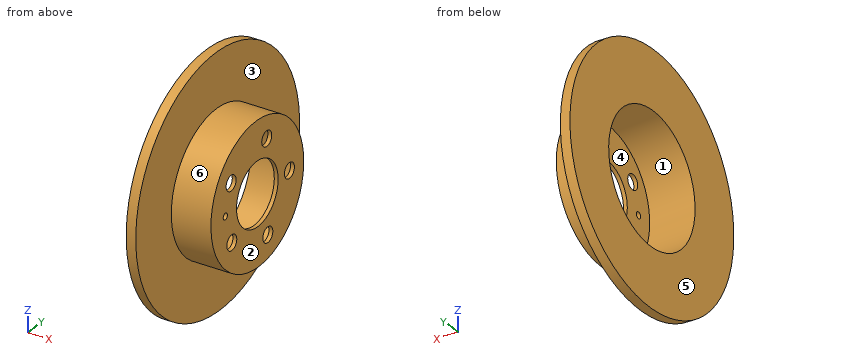
from build123d import *

# Parameters (mm, degrees)
SZKIC1_W                    = 10
SZKIC1_H                    = 128
SZKIC7_R                    = 72.5
DODANIE_WYCI_GNI_CIE1_DEPTH = 41.3
SZKIC8_R                    = 67.5
WYTNIJ_WYCI_GNI_CIE7_DEPTH  = 47.3
WYTNIJ_WYCI_GNI_CIE8_REACH  = 190.148
SZKIC9_R                    = 32.5
WYTNIJ_WYCI_GNI_CIE9_REACH  = 190.148
SZKIC10_R                   = 3.3
SZKIC10_R_2                 = 7.8


with BuildPart() as part:
    # Szkic1 → Obrót1 (revolve)
    with BuildSketch(Plane(origin=(0, 0, 0), x_dir=(1, 0, 0), z_dir=(0, 1, 0)), mode=Mode.PRIVATE) as obr_t1_sk:
        with Locations((5, 64)):
            Rectangle(SZKIC1_W, SZKIC1_H)
    revolve(obr_t1_sk.sketch.rotate(Axis((0, 0, 0), (1, 0, 0)), 180), axis=Axis((0, 0, 0), (1, 0, 0)))

    # Szkic7 → Dodanie-wyciągnięcie1 (add)
    with BuildSketch(Plane(origin=(10, 0, 0), x_dir=(0, 0, -1), z_dir=(1, 0, 0))):
        with Locations(Location((0, 0, 0), (0, 0, 180))):
            Circle(SZKIC7_R)
    extrude(amount=DODANIE_WYCI_GNI_CIE1_DEPTH)

    # Szkic8 → Wytnij-wyciągnięcie7 (cut)
    with BuildSketch(Plane.ZY):
        Circle(SZKIC8_R)
    extrude(amount=-WYTNIJ_WYCI_GNI_CIE7_DEPTH, mode=Mode.SUBTRACT)

    # Szkic9 → Wytnij-wyciągnięcie8 (cut, up to next)
    with BuildSketch(Plane(origin=(51.3, 0, 0), x_dir=(0, 0, -1), z_dir=(1, 0, 0)), mode=Mode.PRIVATE) as wytnij_wyci_gni_cie8_sk1:
        Circle(SZKIC9_R)
    wytnij_wyci_gni_cie8_tool1 = extrude(wytnij_wyci_gni_cie8_sk1.sketch, amount=-WYTNIJ_WYCI_GNI_CIE8_REACH, mode=Mode.PRIVATE) & part.part
    add(wytnij_wyci_gni_cie8_tool1.solids().sort_by_distance((51.3, 0, 0))[0], mode=Mode.SUBTRACT)

    # Szkic10 → Wytnij-wyciągnięcie9 (cut, up to next)
    with BuildSketch(Plane(origin=(51.3, 0, 0), x_dir=(0, 0, -1), z_dir=(1, 0, 0)), mode=Mode.PRIVATE) as wytnij_wyci_gni_cie9_sk1:
        with Locations((0, -50)):
            Circle(SZKIC10_R)
    wytnij_wyci_gni_cie9_tool1 = extrude(wytnij_wyci_gni_cie9_sk1.sketch, amount=-WYTNIJ_WYCI_GNI_CIE9_REACH, mode=Mode.PRIVATE) & part.part
    # Szkic10 → Wytnij-wyciągnięcie9 (cut, up to next)
    with BuildSketch(Plane(origin=(51.3, 0, 0), x_dir=(0, 0, -1), z_dir=(1, 0, 0)), mode=Mode.PRIVATE) as wytnij_wyci_gni_cie9_sk2:
        with Locations((-28.682618124, -40.95494375)):
            Circle(SZKIC10_R_2)
    wytnij_wyci_gni_cie9_tool2 = extrude(wytnij_wyci_gni_cie9_sk2.sketch, amount=-WYTNIJ_WYCI_GNI_CIE9_REACH, mode=Mode.PRIVATE) & part.part
    # Szkic10 → Wytnij-wyciągnięcie9 (cut, up to next)
    with BuildSketch(Plane(origin=(51.3, 0, 0), x_dir=(0, 0, -1), z_dir=(1, 0, 0)), mode=Mode.PRIVATE) as wytnij_wyci_gni_cie9_sk3:
        with Locations((-47.865538925, 14.672227833)):
            Circle(SZKIC10_R_2)
    wytnij_wyci_gni_cie9_tool3 = extrude(wytnij_wyci_gni_cie9_sk3.sketch, amount=-WYTNIJ_WYCI_GNI_CIE9_REACH, mode=Mode.PRIVATE) & part.part
    # Szkic10 → Wytnij-wyciągnięcie9 (cut, up to next)
    with BuildSketch(Plane(origin=(51.3, 0, 0), x_dir=(0, 0, -1), z_dir=(1, 0, 0)), mode=Mode.PRIVATE) as wytnij_wyci_gni_cie9_sk4:
        with Locations((-0.888803437, 50.106011031)):
            Circle(SZKIC10_R_2)
    wytnij_wyci_gni_cie9_tool4 = extrude(wytnij_wyci_gni_cie9_sk4.sketch, amount=-WYTNIJ_WYCI_GNI_CIE9_REACH, mode=Mode.PRIVATE) & part.part
    # Szkic10 → Wytnij-wyciągnięcie9 (cut, up to next)
    with BuildSketch(Plane(origin=(51.3, 0, 0), x_dir=(0, 0, -1), z_dir=(1, 0, 0)), mode=Mode.PRIVATE) as wytnij_wyci_gni_cie9_sk5:
        with Locations((47.327336576, 16.378121814)):
            Circle(SZKIC10_R_2)
    wytnij_wyci_gni_cie9_tool5 = extrude(wytnij_wyci_gni_cie9_sk5.sketch, amount=-WYTNIJ_WYCI_GNI_CIE9_REACH, mode=Mode.PRIVATE) & part.part
    # Szkic10 → Wytnij-wyciągnięcie9 (cut, up to next)
    with BuildSketch(Plane(origin=(51.3, 0, 0), x_dir=(0, 0, -1), z_dir=(1, 0, 0)), mode=Mode.PRIVATE) as wytnij_wyci_gni_cie9_sk6:
        with Locations((30.149814423, -39.900643288)):
            Circle(SZKIC10_R_2)
    wytnij_wyci_gni_cie9_tool6 = extrude(wytnij_wyci_gni_cie9_sk6.sketch, amount=-WYTNIJ_WYCI_GNI_CIE9_REACH, mode=Mode.PRIVATE) & part.part
    add(wytnij_wyci_gni_cie9_tool1.solids().sort_by_distance((51.3, -50, 0))[0], mode=Mode.SUBTRACT)
    add(wytnij_wyci_gni_cie9_tool2.solids().sort_by_distance((51.3, -40.954944, 28.682618))[0], mode=Mode.SUBTRACT)
    add(wytnij_wyci_gni_cie9_tool3.solids().sort_by_distance((51.3, 14.672228, 47.865539))[0], mode=Mode.SUBTRACT)
    add(wytnij_wyci_gni_cie9_tool4.solids().sort_by_distance((51.3, 50.106011, 0.888803))[0], mode=Mode.SUBTRACT)
    add(wytnij_wyci_gni_cie9_tool5.solids().sort_by_distance((51.3, 16.378122, -47.327337))[0], mode=Mode.SUBTRACT)
    add(wytnij_wyci_gni_cie9_tool6.solids().sort_by_distance((51.3, -39.900643, -30.149814))[0], mode=Mode.SUBTRACT)


solid = part.part
Verification items for the finished model (mm, model axes). Face numbers are marked on the shaded views. A direction names the side the tool comes from. Round coordinates to 2 decimals unless told otherwise and drop trailing zeros. Loops run counter-clockwise (first coordinate to the right, second up) from the corner with the lowest first, then second, coordinate; pieces in that order, holes last. Notation, with made-up numbers: (6, 81) - (17, 81) arc R15 cw to (17, 110) - close; hole circle Ø4 at (36, -31.75). An arc over 180 degrees is marked (long way). Answer in a Markdown table with one row per item. Add a question column.
Q1. Section check A-A on y = 0. Enter the section's corners in (x, z), plus the area to 3 significant figures.
Q2. Section check B-B on z = 0. Enter the section's corners in (x, y), plus the area to 3 significant figures.
Q3. Gauge pin test, flat ends, axial feed: pin 1 (2 mm diameter, centred on x = 40, z = -32, fed in from +Y); pin 2 (3 mm diameter, centred on x = 29.5, z = 47, fed in from +Y); pin 3 (25 mm diameter, centred on y = 14.67, z = 47.87, fed in from -X). Record the tip position at first contact, or that the pin passes through.
Q4. Section check D-D on z = -46. Enter the section's corners in (x, y), plus the area to 3 significant figures.
Q5. Material ranges on line 1 (Y direction, x = 49, z = 0); line 2 (Y direction, x = 16.5, z = 0); line 3 (X direction, y = -62, z = 108.5), recorded low to high.
Q6. Release check for a two-part mould opening along Y. For the marked faces 4, 5 and 6 record: pulls with the +Y half, pulls with the -Y half, needs draft (parallel to the pull), parting line crosses it, or undercut.
Q7. Tool access check on the marked faces 1, 2 and 3. Record the directions out of +Z, -Z, +X, -X, +Y, -Y that give a thin tool (end or side, any length) a straight path to the whole face; none if there is none.
Q8. Section check C-C on x = 28. Enter the section's corners in (y, z).
Found:
| question | item | result |
|---|---|---|
| 1 | outline | (0, -128) - (10, -128) - (10, -72.5) - (51.3, -72.5) - (51.3, -32.5) - (47.3, -32.5) - (47.3, -67.5) - (0, -67.5) - close; (0, 67.5) - (47.3, 67.5) - (47.3, 32.5) - (51.3, 32.5) - (51.3, 72.5) - (10, 72.5) - (10, 128) - (0, 128) - close |
| 1 | area | 1,900 mm² |
| 2 | outline | (0, -128) - (10, -128) - (10, -72.5) - (51.3, -72.5) - (51.3, -53.3) - (47.3, -53.3) - (47.3, -67.5) - (0, -67.5) - close; (0, 67.5) - (47.3, 67.5) - (47.3, 57.86) - (51.3, 57.86) - (51.3, 72.5) - (10, 72.5) - (10, 128) - (0, 128) - close; (47.3, -46.7) - (51.3, -46.7) - (51.3, -32.5) - (47.3, -32.5) - close; (47.3, 32.5) - (51.3, 32.5) - (51.3, 42.36) - (47.3, 42.36) - close |
| 2 | area | 1,810 mm² |
| 3 | pin 1 | stops at y = 65.54 |
| 3 | pin 2 | stops at y = 56.44 |
| 3 | pin 3 | stops at x = 47.3 |
| 4 | outline | (0, -119.45) - (10, -119.45) - (10, -56.04) - (51.3, -56.04) - (51.3, 8.69) - (47.3, 8.69) - (47.3, -49.4) - (0, -49.4) - close; (0, 49.4) - (47.3, 49.4) - (47.3, 24.06) - (51.3, 24.06) - (51.3, 56.04) - (10, 56.04) - (10, 119.45) - (0, 119.45) - close |
| 4 | area | 2,280 mm² |
| 5 | line 1 | y = -72.5 to -53.3, -46.7 to -32.5, 32.5 to 42.36, 57.86 to 72.5 |
| 5 | line 2 | y = -72.5 to -67.5, 67.5 to 72.5 |
| 5 | line 3 | x = 0 to 10 |
| 6 | face 4 | undercut |
| 6 | face 5 | needs draft |
| 6 | face 6 | parting line crosses it |
| 7 | face 1 | -X |
| 7 | face 2 | +Z, -Z, +X, +Y, -Y |
| 7 | face 3 | +X |
| 8 | outline | circle Ø145 at (0, 0); hole circle Ø135 at (0, 0) |
